```python
from build123d import *

# Parameters (mm, degrees)
SKETCH1_W           = 101.6
SKETCH1_H           = 57.15
BOSS_EXTRUDE1_DEPTH = 12.7
SKETCH2_R           = 6.35
CUT_EXTRUDE1_DEPTH  = 12.7
SKETCH2_3_R         = 12.7
SKETCH2_3_R_2       = 6.35
CUT_EXTRUDE2_DEPTH  = 2.54
FILLET1_R           = 12.7


with BuildPart() as part:
    # Sketch1 → Boss-Extrude1 (new body)
    with BuildSketch(Plane(origin=(0, 0, 0), x_dir=(1, 0, 0), z_dir=(0, 1, 0))):
        Rectangle(SKETCH1_W, SKETCH1_H)
    extrude(amount=BOSS_EXTRUDE1_DEPTH)

    # Sketch2 → Cut-Extrude1 (cut)
    with BuildSketch(Plane(origin=(0, 12.7, 0), x_dir=(1, 0, 0), z_dir=(0, 1, 0))):
        with Locations((-25.4, 0)):
            Circle(SKETCH2_R)
        with Locations((25.4, 0)):
            Circle(SKETCH2_R)
    extrude(amount=-CUT_EXTRUDE1_DEPTH, mode=Mode.SUBTRACT)

    # Sketch2_3 → Cut-Extrude2 (cut)
    with BuildSketch(Plane(origin=(0, 12.7, 0), x_dir=(1, 0, 0), z_dir=(0, 1, 0))):
        with Locations((-25.4, 0)):
            Circle(SKETCH2_3_R)
        with Locations((-25.4, 0)):
            Circle(SKETCH2_3_R_2, mode=Mode.SUBTRACT)
        with Locations((25.4, 0)):
            Circle(SKETCH2_3_R)
        with Locations((25.4, 0)):
            Circle(SKETCH2_3_R_2, mode=Mode.SUBTRACT)
    extrude(amount=-CUT_EXTRUDE2_DEPTH, mode=Mode.SUBTRACT)

    # Fillet1
    fillet1_edges = [part.edges().sort_by_distance(p)[0] for p in [
        (-50.8, 6.35, 28.575),
        (-50.8, 6.35, -28.575),
        (50.8, 6.35, -28.575),
        (50.8, 6.35, 28.575),
    ]]
    fillet(fillet1_edges, radius=FILLET1_R)


solid = part.part
```
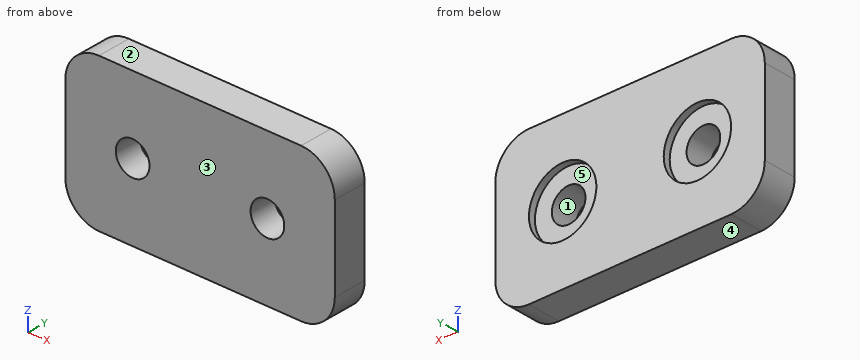
The listing builds one solid part. Answer for the finished solid, in the listing's coordinates (mm). Face numbers are marked on the shaded views. A direction names the side the tool comes from. Round coordinates to 2 decimals unless told otherwise and drop trailing zeros. Loops run counter-clockwise (first coordinate to the right, second up) from the corner with the lowest first, then second, coordinate; pieces in that order, holes last.
Q1. Which of the six approach directions +Z, -Z, +X, -X, +Y, -Y give full straight-line access (tool end or side, diameter ignored) to the marked faces 4 and 5?
Q2. Section D-D, the plane x = 17 is taken. Determine the outline of the cut face in (y, z) (3 decimals), then the cut area to 3 significant figures.
Q3. Section B-B, the plane x = -25.4 is taken. Determine the outline of the cut face in (y, z) (3 decimals), then the cut area to 3 significant figures.
Q4. Section A-A, the plane z = 0 is taken. Determine the outline of the cut face in (x, y).
Q5. For a pull along Z with two mould halves and no side action, classify the marked faces 1, 2 and 3 as released by +Z, released by -Z, zero draft, split by the parting line, or undercut.
Q6. Find the intervals of material crossed by line 1 (X direction, y = 3.75, z = 0); line 2 (X direction, y = 11.8, z = 0); line 3 (Z direction, x = 25.4, y = 5.75) (3 decimals), in increasing order.
Q7. Given pin 1 Ø20.5 at (x, z) = (-25.4, 0) entering from +Y; pin 2 Ø3 at (y, z) = (11, -20) entering from -X, each flat-ended and moving along its own axis, determine where each tip first touches the part or whether it passes through.
Q8. Section C-C, the plane y = 5.5 is taken. Determine the outline of the cut face in (x, z) (3 decimals), then the cut area to 3 significant figures.
Completed:
1. face 4: -Z, +X, -X, +Y, -Y
1. face 5: +Y
2. outline: (0, -28.575) - (12.7, -28.575) - (12.7, -9.525) - (10.16, -9.525) - (10.16, 9.525) - (12.7, 9.525) - (12.7, 28.575) - (0, 28.575) - close
2. area: 677 mm2
3. outline: (0, -28.575) - (12.7, -28.575) - (12.7, -12.7) - (10.16, -12.7) - (10.16, -6.35) - (0, -6.35) - close; (0, 6.35) - (10.16, 6.35) - (10.16, 12.7) - (12.7, 12.7) - (12.7, 28.575) - (0, 28.575) - close
3. area: 532 mm2
4. outline: (-50.8, 0) - (-31.75, 0) - (-31.75, 10.16) - (-38.1, 10.16) - (-38.1, 12.7) - (-50.8, 12.7) - close; (-19.05, 0) - (19.05, 0) - (19.05, 10.16) - (12.7, 10.16) - (12.7, 12.7) - (-12.7, 12.7) - (-12.7, 10.16) - (-19.05, 10.16) - close; (31.75, 0) - (50.8, 0) - (50.8, 12.7) - (38.1, 12.7) - (38.1, 10.16) - (31.75, 10.16) - close
5. face 1: undercut
5. face 2: released by +Z
5. face 3: zero draft
6. line 1: x = -50.8 to -31.75, -19.05 to 19.05, 31.75 to 50.8
6. line 2: x = -50.8 to -38.1, -12.7 to 12.7, 38.1 to 50.8
6. line 3: z = -28.575 to -6.35, 6.35 to 28.575
7. pin 1: stops at y = 10.16
7. pin 2: stops at x = -50.53
8. outline: (-50.8, -15.875) arc R12.7 ccw to (-38.1, -28.575) - (38.1, -28.575) arc R12.7 ccw to (50.8, -15.875) - (50.8, 15.875) arc R12.7 ccw to (38.1, 28.575) - (-38.1, 28.575) arc R12.7 ccw to (-50.8, 15.875) - close; hole circle Ø12.7 at (-25.4, 0); hole circle Ø12.7 at (25.4, 0)
8. area: 5,410 mm2
